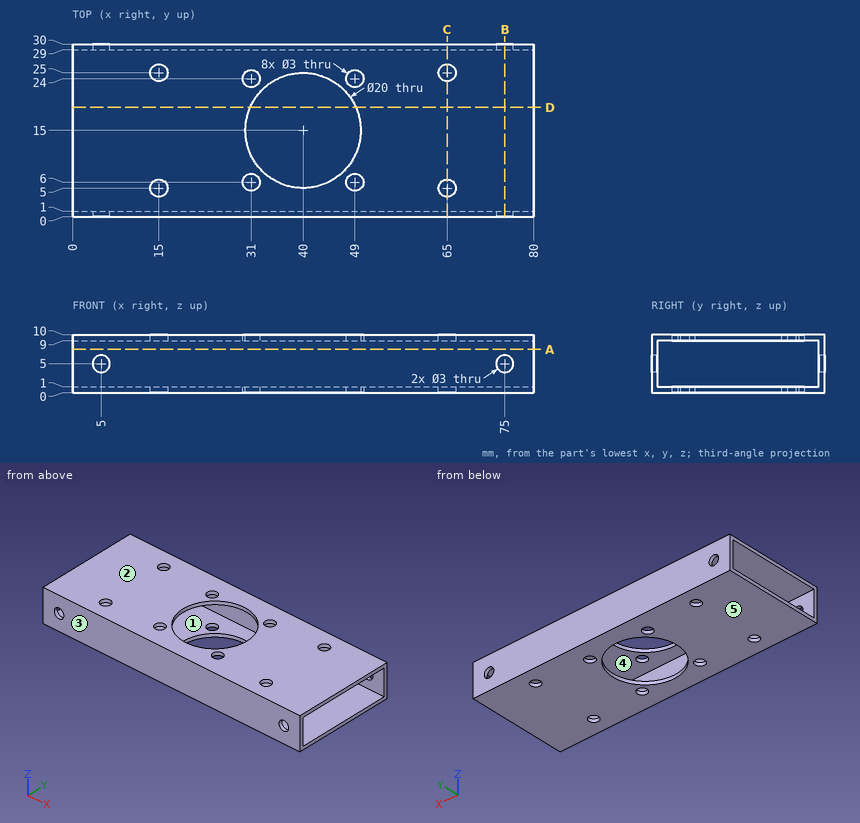
The drawing under review shows one solid part. Ordinate dimensions are in mm from its lowest x, y, z. A direction names the side the tool comes from. Give positions to 0.01 mm unless a question says otherwise; leave off trailing zeros. Write each loop counter-clockwise with the first axis right and the second up, starting at its lowest first coordinate (ties: lowest second). Pieces come first, ordered by that corner, then holes. Notation, with made-up numbers: (-34, -28) - (18, -28) arc R26 cw to (18, -5) - close; hole circle Ø10 at (19, 44). An arc over 180 degrees is marked (long way). Answer in a Markdown table with one row per item. Add a question column.
1. Tool access review of the marked faces 4 and 5: name each direction out of +Z, -Z, +X, -X, +Y, -Y from which nothing blocks a thin tool from reaching the whole face with its end or side.
2. We need section B-B on x = 75. Write out the cut boundary in (y, z), then the cut area to 3 significant figures.
3. Insertion check: P1, Ø2.5, axis at x = 75, z = 5, coming from the +Y side. The pin has a flat end and moves straight along its axis. Give the tip position at first contact, or say it passes through.
4. We need section D-D on y = 19. Write out the cut boundary in (x, z), then the cut area to 3 significant figures.
5. Wall thickness on line 1 along Z through (x, y) = (55, 15.75); line 2 along Y through (x, z) = (63, 7); line 3 along Y through (x, z) = (49, 9.45): over which ranges is each line inside the solid? List them lowest first. Write a range as [from, to].
6. Draft analysis for pull direction Y (two halves, no side actions). For the marked faces 1, 2 and 3, state which applies: +Y half, -Y half, draft (parallel to the pull), parting line (faces both ways), or undercut.
7. We need section C-C on x = 65. Write out the cut boundary in (y, z), then the cut area to 3 significant figures.
8. We need section A-A on z = 7.5. Write out the cut boundary in (x, y).
Ans:
| question | item | result |
|---|---|---|
| 1 | face 4 | +X, -X |
| 1 | face 5 | -Z, +X, -X, +Y, -Y |
| 2 | outline | (0, 0) - (30, 0) - (30, 3.5) - (29, 3.5) - (29, 1) - (1, 1) - (1, 3.5) - (0, 3.5) - close; (0, 6.5) - (1, 6.5) - (1, 9) - (29, 9) - (29, 6.5) - (30, 6.5) - (30, 10) - (0, 10) - close |
| 2 | area | 70.0 mm^2 |
| 3 | P1 | passes through |
| 4 | outline | (0, 0) - (30.83, 0) - (30.83, 1) - (0, 1) - close; (0, 9) - (30.83, 9) - (30.83, 10) - (0, 10) - close; (49.17, 0) - (80, 0) - (80, 1) - (49.17, 1) - close; (49.17, 9) - (80, 9) - (80, 10) - (49.17, 10) - close |
| 4 | area | 123 mm^2 |
| 5 | line 1 | z = [0, 1], [9, 10] |
| 5 | line 2 | y = [0, 1], [29, 30] |
| 5 | line 3 | y = [0, 4.5], [7.5, 10.64], [19.36, 22.5], [25.5, 30] |
| 6 | face 1 | undercut |
| 6 | face 2 | draft |
| 6 | face 3 | -Y half |
| 7 | outline | (0, 0) - (3.5, 0) - (3.5, 1) - (1, 1) - (1, 9) - (3.5, 9) - (3.5, 10) - (0, 10) - close; (6.5, 0) - (23.5, 0) - (23.5, 1) - (6.5, 1) - close; (6.5, 9) - (23.5, 9) - (23.5, 10) - (6.5, 10) - close; (26.5, 0) - (30, 0) - (30, 10) - (26.5, 10) - (26.5, 9) - (29, 9) - (29, 1) - (26.5, 1) - close |
| 7 | area | 64.0 mm^2 |
| 8 | outline | (0, 0) - (80, 0) - (80, 1) - (0, 1) - close; (0, 29) - (80, 29) - (80, 30) - (0, 30) - close |
